```python
from build123d import *

# Parameters (mm, degrees)
AXLE_BASE_SKETCH_R     = 15.5
AXLE_DEPTH             = 93.5
GUARD_BASE_R           = 25
GUARD_DEPTH            = 5
INNER_AXLE_HOLE_BASE_R = 10
INNER_AXLE_HOLE_DEPTH  = 99.5
BEND_ROOM_BASE_W       = 1.5
BEND_ROOM_BASE_H       = 50
BEND_ROOM_1_DEPTH      = 36
BEND_ROOM_2_COUNT      = 2
BEND_ROOM_2_ANGLE      = 90
CHAMFER1_SIZE          = 4


with BuildPart() as part:
    # Axle base sketch → Axle (new body)
    with BuildSketch(Plane.XY):
        Circle(AXLE_BASE_SKETCH_R)
    extrude(amount=AXLE_DEPTH)

    # Guard base → Guard (add)
    with BuildSketch(Plane(origin=(0, 0, 0), x_dir=(-1, 0, 0), z_dir=(0, 0, -1))):
        Circle(GUARD_BASE_R)
    extrude(amount=GUARD_DEPTH)

    # Inner axle hole base → Inner axle hole (cut, through all)
    with BuildSketch(Plane.XY.offset(93.5)):
        Circle(INNER_AXLE_HOLE_BASE_R)
    extrude(amount=-INNER_AXLE_HOLE_DEPTH, mode=Mode.SUBTRACT)

    # Mate ring base → Mate rings (revolve)
    with BuildSketch(Plane(origin=(0, 0, 0), x_dir=(1, 0, 0), z_dir=(0, 1, 0))):
        Polygon((15.5, -93.5), (16.25, -92.75), (16.25, -92), (15.5, -91.25), align=None)
        Polygon((15.5, -87.75), (16.25, -87), (16.25, -86.25), (15.5, -85.5), align=None)
    revolve(axis=Axis((0, 0, 0), (0, 0, -1)))

    # Bend room base → Bend room 1 (cut)
    with BuildSketch(Plane.XY.offset(93.5)):
        Rectangle(BEND_ROOM_BASE_W, BEND_ROOM_BASE_H)
    bend_room_1 = extrude(amount=-BEND_ROOM_1_DEPTH, mode=Mode.SUBTRACT)

    # Bend room 2: Bend room 1 ×2 about axis
    bend_room_2_axis = Axis((0, 0, 0), (0, 0, -1))
    for i in range(1, BEND_ROOM_2_COUNT):
        add(bend_room_1.rotate(bend_room_2_axis, i * BEND_ROOM_2_ANGLE / (BEND_ROOM_2_COUNT - 1)), mode=Mode.SUBTRACT)

    # Chamfer1
    chamfer1_edges = [part.edges().sort_by_distance(p)[0] for p in [
        (25, 0, 0),
    ]]
    chamfer(chamfer1_edges, length=CHAMFER1_SIZE)


solid = part.part
```
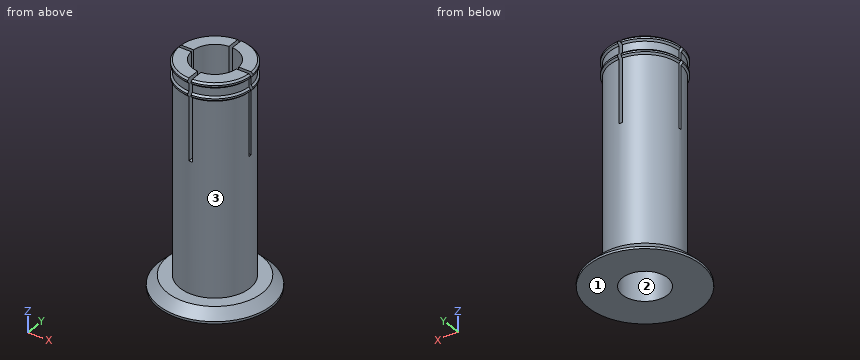
Verification items for the finished model (mm, model axes). Face numbers are marked on the shaded views. Coordinates: 2 decimals unless noted, no trailing zeros. Write each loop counter-clockwise with the first axis right and the second up, starting at its lowest first coordinate (ties: lowest second). Pieces come first, ordered by that corner, then holes. Notation, with made-up numbers: (22, -3) - (40, -3) arc R4 cw to (40, 2) - close; hole circle Ø2 at (85.25, -19). An arc over 180 degrees is marked (long way). Write item = value, one per line.
Q1. Material ranges on L1, parallel to X at y = 0, z = 48.5; L2, parallel to Z at x = 10, y = -12; L3, parallel to Z at x = -19.5, y = 6.5, recorded low to high. Write a range as from..to.
Answer:
L1 = -15.5..-10, 10..15.5
L2 = -5..0, 85.62..87.63, 91.37..93.38
L3 = -5..0
Q2. Cross-section at B-B (z = 26.5). Enter the section's corners in (x, y).
Answer:
outline = circle Ø31 at (0, 0); hole circle Ø20 at (0, 0)
Q3. Cross-section at A-A (z = 66). Enter the section's corners in (x, y), plus the area to 3 significant figures.
Answer:
outline = (-15.48, -0.75) arc R15.5 ccw to (-0.75, -15.48) - (-0.75, -9.97) arc R10 cw to (-9.97, -0.75) - close; (-15.48, 0.75) - (-9.97, 0.75) arc R10 cw to (-0.75, 9.97) - (-0.75, 15.48) arc R15.5 ccw to start; (0.75, -15.48) arc R15.5 ccw to (15.48, -0.75) - (9.97, -0.75) arc R10 cw to (0.75, -9.97) - close; (0.75, 9.97) arc R10 cw to (9.97, 0.75) - (15.48, 0.75) arc R15.5 ccw to (0.75, 15.48) - close
area = 408 mm²
Q4. Mould release check, pull along Y, two halves, no side actions. Record for the marked faces 1, 2 and 3: released by +Y, released by -Y, zero draft, split by the parting line, or undercut.
Answer:
face_1 = zero draft
face_2 = undercut
face_3 = split by the parting line
Q5. Go/stop test with flat-tipped pins: pin 1 Ø7 at (y, z) = (-12, 79.5) entering from +X; pin 2 Ø0.5 at (x, y) = (12, 0) entering from +Z; pin 3 Ø1.7 at (x, y) = (-12.5, 0) entering from +Z; pin 4 Ø12 at (x, z) = (14, 45) entering from -Y. Record where each tip stops, or that it passes through.
Answer:
pin_1 = 12.96
pin_2 = 57.5
pin_3 = 93.5
pin_4 = -13.28
